Autodesk Inventor part; units mm, degrees
ref_plane "YZ Plane" through (0, 0, 0) normal (1, 0, 0) x (0, 1, 0)
ref_plane "XZ Plane" through (0, 0, 0) normal (0, 1, 0) x (-1, 0, 0)
ref_plane "XY Plane" through (0, 0, 0) normal (0, 0, 1) x (1, 0, 0)
sketch "Skizze1" plane through (0, 0, 0) normal (0, 1, 0) x (-1, 0, 0)
  circle A0 centre (0, 0) radius 11.5
  dimension "d0" = 23
extrude "Extrusion1" add sketch "Skizze1" along normal blind 55
sketch "Skizze2" plane through (0, 55, 0) normal (0, 1, 0) x (1, 0, 0)
  circle A0 centre (0, 0) radius 7
  dimension "d3" = 14
extrude "Extrusion2" cut sketch "Skizze2" against normal blind 25
sketch "Skizze3" plane through (0, 55, 0) normal (0, 1, 0) x (1, 0, 0)
  line L0 (12.5, -2.25) -> (-12.5, -2.25)
  line L1 (-12.5, -2.25) -> (-12.5, 2.25)
  line L2 (-12.5, 2.25) -> (12.5, 2.25)
  line L3 (12.5, 2.25) -> (12.5, -2.25)
  line L4 (-17.5, 0) -> (17.5, 0)
  line L5 (0, 16.1) -> (0, -16.1)
  point P0 (0, 0)
  dimension "d6" = 4.5
  dimension "d7" = 25
extrude "Extrusion3" cut sketch "Skizze3" against normal blind 20
sketch "Skizze4" plane through (0, 0, 0) normal (0, -1, 0) x (1, 0, 0)
  circle A0 centre (0, 0) radius 7.5
  line L0 (-7.0711, -2.5) -> (-9.5, -2.5)
  line L1 (-9.5, -2.5) -> (-9.5, 2.5)
  line L2 (-9.5, 2.5) -> (-7.0711, 2.5)
  line L3 (-7.0711, 2.5) -> (-7.0711, -2.5)
  line L4 (-16.1, 0) -> (16.1, 0)
  point P0 (7.5, 0)
  point P1 (-7.0711, 2.5)
  dimension "d10" = 15
  dimension "d12" = 17
  dimension "d13" = 5
extrude "Extrusion4" cut sketch "Skizze4" against normal blind 25
properties part number "Honigfschleuder Motorkupplung"
Design review of the part built by this model. Coordinates are the model's own, in mm. A direction names the side the tool comes from. Round coordinates to 2 decimals unless told otherwise and drop trailing zeros. Loops run counter-clockwise (first coordinate to the right, second up) from the corner with the lowest first, then second, coordinate; pieces in that order, holes last. Notation, with made-up numbers: (-23, 25.5) -> (-2, 25.5) arc R24 ccw to (-2, 42.5) -> close; hole circle Ø1 at (28, 81.25). An arc over 180 degrees is marked (long way). Use one line per item in the form item = value. Start each with the question number.
Q1. We need section D-D on y = 31.5. Give the boundary of the cut face in (x, z), then the cut area to 3 significant figures.
Q2. Wall thickness on line 1 along Z through (x, y) = (0, 48.75); line 2 along Z through (x, y) = (0, 5); line 3 along X through (y, z) = (17, 0): over which ranges is each line inside the solid? List them lowest first. Write a range as [from, to].
Q3. For pin 1 Ø12 at (x, z) = (8, -3.5) entering from -Y; pin 2 Ø2.5 at (x, y) = (-8, 45.5) entering from +Z; pin 3 Ø3 at (y, z) = (41.5, 4.5) entering from -X; pin 4 Ø5 at (x, z) = (2.5, -1) entering from +Y, all flat-tipped, find the tip position at first contact; note any pin that passes through.
Q4. We need section B-B on z = 0. Give the boundary of the cut face in (x, y), then the cut area to 3 significant figures.
Q5. Draft analysis for pull direction Z (two halves, no side actions). For faces 4 (the face through (9, 45, -2.25)), 5 (the face through (0, 55, -8)), 6 (the face through (-10.97, 27.12, -3.45)), state which applies: +Z half, -Z half, draft (parallel to the pull), parting line (faces both ways), or undercut.
Q6. We need section A-A on y = 44.5. Give the boundary of the cut face in (x, z).
Q7. Machinability: for faces 1 (the face through (0, 30, 0)), 2 (the face through (9, 45, 2.25)), 3 (the face through (-9.5, 12, 0)), which of the approach directions +Z, -Z, +X, -X, +Y, -Y give a long, thin tool a straight path to every point of the face, cutting with its end or side? Answer none if there is none.
Q8. We need section C-C on x = 0. Give the boundary of the cut face in (y, z), then the cut area to 3 significant figures.
Calculated:
q1.outline = circle Ø23 at (0, 0); hole circle Ø14 at (0, 0)
q1.area = 262 mm²
q2.line_1 = [-11.5, -7], [7, 11.5]
q2.line_2 = [-11.5, -7.5], [7.5, 11.5]
q2.line_3 = [-11.5, -9.5], [7.5, 11.5]
q3.pin_1 = 0
q3.pin_2 = 9.31
q3.pin_3 = -11.1
q3.pin_4 = 30
q4.outline = (-11.5, 0) -> (-9.5, 0) -> (-9.5, 25) -> (7.5, 25) -> (7.5, 0) -> (11.5, 0) -> (11.5, 35) -> (7, 35) -> (7, 30) -> (-7, 30) -> (-7, 35) -> (-11.5, 35) -> close
q4.area = 310 mm²
q5.face_4 = undercut
q5.face_5 = draft
q5.face_6 = parting line
q6.outline = (-11.28, -2.25) arc R11.5 ccw to (11.28, -2.25) -> (6.63, -2.25) arc R7 cw to (-6.63, -2.25) -> close; (-11.28, 2.25) -> (-6.63, 2.25) arc R7 cw to (6.63, 2.25) -> (11.28, 2.25) arc R11.5 ccw to start
q7.face_1 = +Y
q7.face_2 = +X, -X, +Y
q7.face_3 = -Y
q8.outline = (0, -11.5) -> (55, -11.5) -> (55, -7) -> (30, -7) -> (30, 7) -> (55, 7) -> (55, 11.5) -> (0, 11.5) -> (0, 7.5) -> (25, 7.5) -> (25, -7.5) -> (0, -7.5) -> close
q8.area = 540 mm²
